Can you work these out from the model? Positions are in its coordinate system, mm. Face numbers are marked on the shaded views. A direction names the side the tool comes from. Give positions to 0.01 mm unless a question says otherwise; leave off trailing zeros. Order: outer loops, then holes, each group sorted by start corner. A loop starts at its lowest first (then second) coordinate and runs counter-clockwise, first axis right, second up.
Item 1: I'm going to push flat-ended pins straight in: pin 1 Ø14 at (y, z) = (-12.84, 21.66) entering from +X; pin 2 Ø8.5 at (x, y) = (4.5, -51) entering from +Z. Where does each tip first touch, or does it pass through?
Item 2: If we mould it in two halves opening along Y, with no side actions, what happens to the marked faces 4, 5, 6 and 7? For each: +Y half, -Y half, draft (parallel to the pull), parting line (faces both ways), or undercut.
Item 3: I want a section at A-A, the plane y = 12.5. Write out the boundary of the cut face in (x, z).
Item 4: I want a section at D-D, the plane z = 6.5. Write out the boundary of the cut face in (x, y).
Item 5: Which directions (+Z, -Z, +X, -X, +Y, -Y) give clear straight access to the entire face, cutting with the end or side of a thin tool? Please do the marked faces 1, 2 and 3.
Item 6: I want a section at C-C, the plane z = 40.5. Write out the boundary of the cut face in (x, y).
Item 7: If I drill on line 1 along X through (y, z) = (-1.5, 32); line 2 along Y through (x, z) = (68, 47); line 3 along X through (y, z) = (32, 35), over which ranges is the centre line in solid material (lowest first)?
Item 8: I want a section at B-B, the plane x = 26. Write out the boundary of the cut face in (y, z), then the cut area to 3 significant figures.
```python
from build123d import *

# Parameters (mm, degrees)
F0_W     = 163.8257876039
F0_H     = 100.1764573157
F0_W_2   = 141.6816487908
F0_H_2   = 72.07223773
F1_DEPTH = 50.038
F2_W     = 85.1234197617
F2_H     = 20.8614202117
F3_DEPTH = 132.842
F4_R     = 8.6739070384
F5_DEPTH = 191.516


with BuildPart() as f1:
    # F0 (on Top) → F1 (new body)
    with BuildSketch(Plane.XY):
        with Locations((10.3731565177, -12.8415655345)):
            Rectangle(F0_W, F0_H)
        with Locations((6.2276907265, -9.8548047245)):
            Rectangle(F0_W_2, F0_H_2, mode=Mode.SUBTRACT)
    extrude(amount=F1_DEPTH)

    # F2 (on face) → F3 (cut)
    with BuildSketch(Plane.XZ.offset(62.9297941923)):
        with Locations((10.2989450097, 39.6072898942)):
            Rectangle(F2_W, F2_H)
    extrude(amount=-F3_DEPTH, mode=Mode.SUBTRACT)

    # F4 (on face) → F5 (cut)
    with BuildSketch(Plane(origin=(-71.5397372842, 0, 0), x_dir=(0, -1, 0), z_dir=(-1, 0, 0))):
        with Locations((12.8415655345, 21.6568429023)):
            Circle(F4_R)
    extrude(amount=-F5_DEPTH, mode=Mode.SUBTRACT)


solid = f1.part
```
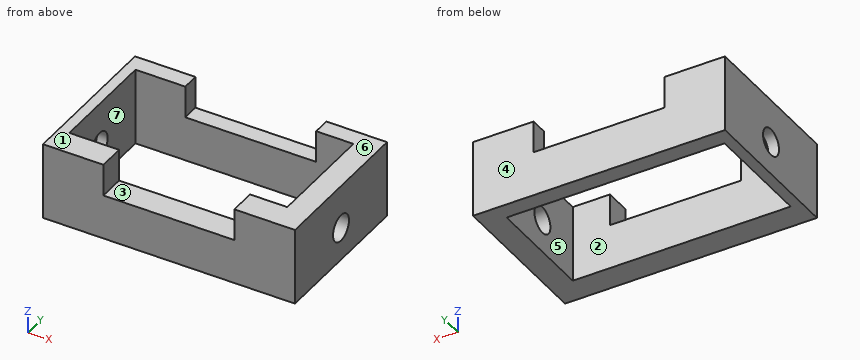
Results list:
1. pin 1: passes through
1. pin 2: stops at z = 29.18
2. face 4: +Y half
2. face 5: undercut
2. face 6: draft
2. face 7: undercut
3. outline: (-71.54, 0) - (-64.61, 0) - (-64.61, 50.04) - (-71.54, 50.04) - close; (77.07, 0) - (92.29, 0) - (92.29, 50.04) - (77.07, 50.04) - close
4. outline: (-71.54, -62.93) - (92.29, -62.93) - (92.29, 37.25) - (-71.54, 37.25) - close; hole (-64.61, -45.89) - (77.07, -45.89) - (77.07, 26.18) - (-64.61, 26.18) - close
5. face 1: +Z, +X, -X, +Y, -Y
5. face 2: +Z, -Z
5. face 3: +Z, +Y, -Y
6. outline: (-71.54, -62.93) - (-32.26, -62.93) - (-32.26, -45.89) - (-64.61, -45.89) - (-64.61, 26.18) - (-32.26, 26.18) - (-32.26, 37.25) - (-71.54, 37.25) - close; (52.86, -62.93) - (92.29, -62.93) - (92.29, 37.25) - (52.86, 37.25) - (52.86, 26.18) - (77.07, 26.18) - (77.07, -45.89) - (52.86, -45.89) - close
7. line 1: x = -71.54 to -64.61, 77.07 to 92.29
7. line 2: y = -62.93 to -45.89, 26.18 to 37.25
7. line 3: x = -71.54 to -32.26, 52.86 to 92.29
8. outline: (-62.93, 0) - (-45.89, 0) - (-45.89, 29.18) - (-62.93, 29.18) - close; (26.18, 0) - (37.25, 0) - (37.25, 29.18) - (26.18, 29.18) - close
8. area: 820 mm2
